from build123d import *

# Parameters (mm, degrees)
F1_DEPTH = 500
F3_DEPTH = 23.191775822
F4_W     = 105
F4_H     = 220
F4_R     = 3.5
F4_R_2   = 4
F5_DEPTH = 6.001
F6_R     = 4
F7_DEPTH = 6.001


with BuildPart() as f1:
    # F0 (on Right) → F1 (new body)
    with BuildSketch(Plane.YZ):
        Polygon((700, 0), (0, 0), (-98.4807753012, 17.3648177667), (-99.5226643672, 11.4559712486), (0, -6), (700, -6), align=None)
    extrude(amount=F1_DEPTH)

    # F2 (on face) → F3 (cut, through all)
    with BuildSketch(Plane(origin=(0, 0, 0), x_dir=(1, 0, 0), z_dir=(0, 0.1736481777, 0.984807753))):
        with BuildLine():
            Line((0, -100), (50, -100))
            ThreePointArc((50, -100), (14.6446609407, -85.3553390593), (0, -50))
            Line((0, -50), (0, -100))
        make_face()
        with BuildLine():
            ThreePointArc((500, -50), (485.3553390593, -85.3553390593), (450, -100))
            Line((450, -100), (500, -100))
            Line((500, -100), (500, -50))
        make_face()
    extrude(amount=-F3_DEPTH, mode=Mode.SUBTRACT)

    # F4 (on face) → F5 (cut, through all)
    with BuildSketch(Plane.XY):
        with Locations((102.5, 540)):
            Rectangle(F4_W, F4_H)
        with Locations((35, 500)):
            Circle(F4_R)
        with Locations((15, 500)):
            Circle(F4_R)
        with Locations((35, 580)):
            Circle(F4_R)
        with Locations((15, 580)):
            Circle(F4_R)
        with Locations((190, 500)):
            Circle(F4_R)
        with Locations((170, 500)):
            Circle(F4_R)
        with Locations((190, 580)):
            Circle(F4_R)
        with Locations((170, 580)):
            Circle(F4_R)
        with Locations((465, 500)):
            Circle(F4_R)
        with Locations((485, 500)):
            Circle(F4_R)
        with Locations((485, 580)):
            Circle(F4_R)
        with Locations((310, 500)):
            Circle(F4_R)
        with Locations((465, 580)):
            Circle(F4_R)
        with Locations((330, 500)):
            Circle(F4_R)
        with Locations((330, 580)):
            Circle(F4_R)
        with Locations((310, 580)):
            Circle(F4_R)
        with Locations((397.5, 540)):
            Rectangle(F4_W, F4_H)
        with Locations((30, 30)):
            Circle(F4_R_2)
        with Locations((470, 30)):
            Circle(F4_R_2)
    extrude(amount=-F5_DEPTH, mode=Mode.SUBTRACT)

    # F6 (on face) → F7 (cut, through all)
    with BuildSketch(Plane.XY):
        with Locations((23, 100)):
            Circle(F6_R)
        with Locations((40.6847405975, 82.3152594025)):
            Circle(F6_R)
        with Locations((23, 659.3152594025)):
            Circle(F6_R)
        with Locations((40.6847405975, 677)):
            Circle(F6_R)
        with Locations((459.3152594025, 677)):
            Circle(F6_R)
        with Locations((477, 659.3152594025)):
            Circle(F6_R)
        with Locations((477, 100)):
            Circle(F6_R)
        with Locations((459.3152594025, 82.3152594025)):
            Circle(F6_R)
    extrude(amount=-F7_DEPTH, mode=Mode.SUBTRACT)


solid = f1.part
Input: part model. Units: mm. Frame: model coordinates. A direction names the side the tool comes from. Coordinates: 2 decimals unless noted, no trailing zeros. Loops run counter-clockwise (first coordinate to the right, second up) from the corner with the lowest first, then second, coordinate; pieces in that order, holes last. Notation, with made-up numbers: (86.5, -31) - (143.5, -31) arc R30 cw to (143.5, 7) - close; hole circle Ø9 at (-2.75, 59.5). An arc over 180 degrees is marked (long way). Answer in a Markdown table with one row per item. Add a question column.
Item 1: Access query for faces 1 (the flat face through (246, 345, -6)), 2 (the flat face through (246, 355, 0)). Directions: +Z, -Z, +X, -X, +Y, -Y. A direction counts if a zero-diameter tool reaches every point of the face in a straight line with its end or side. Return the directions, or none.
Item 2: Contact query for flat-ended pins moving along their axis: P1, Ø12, axis at x = 331.5, y = 384, coming from the +Z side; P2, Ø6.5, axis at x = 477, y = 659.32, coming from the +Z side. Output: stop coordinate, or through.
Item 3: Section query C-C on x = 245.5. Return the cut outline in (y, z), then the cut area to 3 significant figures.
Item 4: Section query A-A on y = 547. Return the cut outline in (x, z), then the cut area to 3 significant figures.
Item 5: Line query: line 1 along X through (y, z) = (540, -2.25); line 2 along Z through (x, y) = (38, 109); line 3 along Z through (x, y) = (254.5, -27). Output: solid intervals per line, ascending. Write a range as [from, to].
Item 6: Section query D-D on y = 267.5. Return the cut outline in (x, z).
Item 7: Section query B-B on x = 112.5. Return the cut outline in (y, z).
Recorded:
| question | item | result |
|---|---|---|
| 1 | face 1 | -Z, +X, -X, +Y, -Y |
| 1 | face 2 | +Z, +X, -X, +Y |
| 2 | P1 | z = 0 |
| 2 | P2 | through |
| 3 | outline | (-99.52, 11.46) - (0, -6) - (700, -6) - (700, 0) - (0, 0) - (-98.48, 17.36) - close |
| 3 | area | 4,800 mm^2 |
| 4 | outline | (0, -6) - (50, -6) - (50, 0) - (0, 0) - close; (155, -6) - (345, -6) - (345, 0) - (155, 0) - close; (450, -6) - (500, -6) - (500, 0) - (450, 0) - close |
| 4 | area | 1,740 mm^2 |
| 5 | line 1 | [0, 50], [155, 345], [450, 500] |
| 5 | line 2 | [-6, 0] |
| 5 | line 3 | [-1.26, 4.76] |
| 6 | outline | (0, -6) - (500, -6) - (500, 0) - (0, 0) - close |
| 7 | outline | (-99.52, 11.46) - (0, -6) - (430, -6) - (430, 0) - (0, 0) - (-98.48, 17.36) - close; (650, -6) - (700, -6) - (700, 0) - (650, 0) - close |
